Work out the finished part from the listing and answer in its coordinate system (mm). A direction names the side the tool comes from. Round coordinates to 2 decimals unless told otherwise and drop trailing zeros. Loops run counter-clockwise (first coordinate to the right, second up) from the corner with the lowest first, then second, coordinate; pieces in that order, holes last.
```python
from build123d import *

# Parameters (mm, degrees)
ESQUISSE1_R             = 12.5
BOSS_EXTRU_1_DEPTH      = 25
BOSS_EXTRU_2_DEPTH      = 40
CONG_1_R                = 10
ESQUISSE5_W             = 15
ESQUISSE5_H             = 25
BOSS_EXTRU_3_DEPTH      = 50
BOSS_EXTRU_4_DEPTH      = 5
BOSS_EXTRU_4_DEPTH_BACK = 35
ESQUISSE6_W             = 40
ESQUISSE6_H             = 40
CONG_2_R                = 10
CONG_3_R                = 10
ESQUISSE8_R             = 7.5
ENL_V_MAT_EXTRU_2_DEPTH = 20
CONG_4_R                = 10


with BuildPart() as part:
    # Esquisse1 → Boss.-Extru.1 (new body)
    with BuildSketch(Plane.XY):
        Circle(ESQUISSE1_R)
    extrude(amount=BOSS_EXTRU_1_DEPTH)

    # Esquisse2 → Boss.-Extru.2 (add)
    with BuildSketch(Plane.XY.offset(25)):
        with BuildLine():
            Line((-10, 20), (10, 20))
            ThreePointArc((10, 20), (17.071067812, 17.071067812), (20, 10))
            Line((20, 10), (20, -10))
            ThreePointArc((20, -10), (17.071067812, -17.071067812), (10, -20))
            Line((10, -20), (-10, -20))
            ThreePointArc((-10, -20), (-17.071067812, -17.071067812), (-20, -10))
            Line((-20, -10), (-20, 10))
            ThreePointArc((-20, 10), (-17.071067812, 17.071067812), (-10, 20))
        make_face()
    extrude(amount=BOSS_EXTRU_2_DEPTH)

    # Congé1
    cong_1_edges = [part.edges().sort_by_distance(p)[0] for p in [
        (0, 20, 65),
        (-17.071067812, 17.071067812, 65),
        (-20, 0, 65),
        (-17.071067812, -17.071067812, 65),
        (0, -20, 65),
        (17.071067812, -17.071067812, 65),
        (20, 0, 65),
        (17.071067812, 17.071067812, 65),
    ]]
    fillet(cong_1_edges, radius=CONG_1_R)

    # Esquisse5 → Boss.-Extru.3 (add)
    with BuildSketch(Plane.XZ.offset(20)):
        with Locations((0, 40)):
            Rectangle(ESQUISSE5_W, ESQUISSE5_H)
    extrude(amount=BOSS_EXTRU_3_DEPTH)

    # Esquisse6 → Boss.-Extru.4 (add, two sides: drawn at the far end of the back side and taken through both)
    with BuildSketch(Plane(origin=(0, 0, 27.5), x_dir=(-1, 0, 0), z_dir=(0, 0, -1)).offset(-BOSS_EXTRU_4_DEPTH_BACK)):
        with Locations((0, -90)):
            Rectangle(ESQUISSE6_W, ESQUISSE6_H)
    extrude(amount=BOSS_EXTRU_4_DEPTH + BOSS_EXTRU_4_DEPTH_BACK)

    # Congé2
    cong_2_edges = [part.edges().sort_by_distance(p)[0] for p in [
        (-20, -110, 42.5),
        (0, -110, 62.5),
        (20, -110, 42.5),
        (0, -110, 22.5),
    ]]
    fillet(cong_2_edges, radius=CONG_2_R)

    # Congé3
    # the kernel refuses this fillet: 10 mm, written as the material it takes off along each edge
    with BuildSketch(Plane(origin=(10, -100, 32.5), x_dir=(1, 0, 0), z_dir=(0, 0, -1))) as cong_3_piece_1_section:
        Polygon((0, 0), (CONG_3_R, 0), (CONG_3_R, CONG_3_R), (0, CONG_3_R), align=None)
    cong_3_piece_1 = extrude(amount=CONG_3_R, mode=Mode.PRIVATE)
    cong_3_piece_1 = cong_3_piece_1 - Plane(origin=(10, -100, 32.5), x_dir=(-0.7071067811865475, 0.7071067811865475, 0), z_dir=(0, 0, -1)) * Sphere(CONG_3_R, mode=Mode.PRIVATE)
    add(cong_3_piece_1, mode=Mode.SUBTRACT)
    with BuildSketch(Plane(origin=(-10, -100, 32.5), x_dir=(0, 0, -1), z_dir=(-1, 0, 0))) as cong_3_piece_2_section:
        Polygon((0, 0), (CONG_3_R, 0), (CONG_3_R, CONG_3_R), (0, CONG_3_R), align=None)
    cong_3_piece_2 = extrude(amount=CONG_3_R, mode=Mode.PRIVATE)
    cong_3_piece_2 = cong_3_piece_2 - Plane(origin=(-10, -100, 32.5), x_dir=(0, 0.7071067811865475, 0.7071067811865475), z_dir=(-1, 0, 0)) * Sphere(CONG_3_R, mode=Mode.PRIVATE)
    add(cong_3_piece_2, mode=Mode.SUBTRACT)
    with BuildSketch(Plane(origin=(10, -100, 52.5), x_dir=(1, 0, 0), z_dir=(0, 0, 1))) as cong_3_piece_3_section:
        Polygon((0, 0), (CONG_3_R, 0), (CONG_3_R, -CONG_3_R), (0, -CONG_3_R), align=None)
    cong_3_piece_3 = extrude(amount=CONG_3_R, mode=Mode.PRIVATE)
    cong_3_piece_3 = cong_3_piece_3 - Plane(origin=(10, -100, 52.5), x_dir=(-0.7071067811865475, 0.7071067811865475, 0), z_dir=(0, 0, 1)) * Sphere(CONG_3_R, mode=Mode.PRIVATE)
    add(cong_3_piece_3, mode=Mode.SUBTRACT)
    with BuildSketch(Plane(origin=(-10, -100, 52.5), x_dir=(0, 0, 1), z_dir=(-1, 0, 0))) as cong_3_piece_4_section:
        Polygon((0, 0), (CONG_3_R, 0), (CONG_3_R, -CONG_3_R), (0, -CONG_3_R), align=None)
    cong_3_piece_4 = extrude(amount=CONG_3_R, mode=Mode.PRIVATE)
    cong_3_piece_4 = cong_3_piece_4 - Plane(origin=(-10, -100, 52.5), x_dir=(0, 0.7071067811865475, -0.7071067811865475), z_dir=(-1, 0, 0)) * Sphere(CONG_3_R, mode=Mode.PRIVATE)
    add(cong_3_piece_4, mode=Mode.SUBTRACT)
    with BuildSketch(Plane(origin=(20, -45, 62.5), x_dir=(-1, 0, 0), z_dir=(0, -1, 0)), Plane(origin=(-20, -100, 22.5), x_dir=(0, 0, 1), z_dir=(0, 1, 0))) as cong_3_piece_5:
        with BuildLine():
            CenterArc((CONG_3_R, CONG_3_R), CONG_3_R, 180, 90)
            Line((0, CONG_3_R), (0, 0))
            Line((0, 0), (CONG_3_R, 0))
        make_face()
    extrude(amount=55, mode=Mode.SUBTRACT)
    with BuildSketch(Plane(origin=(20, -45, 22.5), x_dir=(-1, 0, 0), z_dir=(0, -1, 0)), Plane(origin=(-20, -100, 62.5), x_dir=(0, 0, -1), z_dir=(0, 1, 0))) as cong_3_piece_6:
        with BuildLine():
            CenterArc((CONG_3_R, -CONG_3_R), CONG_3_R, 90, 90)
            Line((0, -CONG_3_R), (0, 0))
            Line((0, 0), (CONG_3_R, 0))
        make_face()
    extrude(amount=55, mode=Mode.SUBTRACT)

    # Esquisse8 → Enlèv. mat.-Extru.2 (cut)
    with BuildSketch(Plane(origin=(0, 0, 22.5), x_dir=(-1, 0, 0), z_dir=(0, 0, -1))):
        with Locations((0, -85)):
            Circle(ESQUISSE8_R)
    extrude(amount=-ENL_V_MAT_EXTRU_2_DEPTH, mode=Mode.SUBTRACT)

    # Congé4
    # the kernel refuses this fillet: 10 mm, written as the material it takes off along each edge
    with BuildSketch(Plane(origin=(-10, -70, 52.5), x_dir=(0, 0, 1), z_dir=(1, 0, 0))) as cong_4_piece_1:
        with BuildLine():
            CenterArc((10 - CONG_4_R, CONG_4_R), CONG_4_R, 270, 90)
            Line((10 - CONG_4_R, 0), (10, 0))
            Line((10, 0), (10, CONG_4_R))
        make_face()
    revolve(axis=Axis((-10, -70, 52.5), (0, -1, 0)), revolution_arc=90, mode=Mode.SUBTRACT)
    with BuildSketch(Plane(origin=(-10, -70, 62.5), x_dir=(0, 0, -1), z_dir=(1, 0, 0)), Plane(origin=(20, -70, 52.5), x_dir=(-1, 0, 0), z_dir=(0, 0, -1))) as cong_4_piece_2:
        with BuildLine():
            CenterArc((CONG_4_R, -CONG_4_R), CONG_4_R, 90, 90)
            Line((0, -CONG_4_R), (0, 0))
            Line((0, 0), (CONG_4_R, 0))
        make_face()
    extrude(amount=20, mode=Mode.SUBTRACT)
    with BuildSketch(Plane(origin=(10, -70, 52.5), x_dir=(0, 0, 1), z_dir=(-1, 0, 0))) as cong_4_piece_3:
        with BuildLine():
            CenterArc((10 - CONG_4_R, -CONG_4_R), CONG_4_R, 0, 90)
            Line((10, -CONG_4_R), (10, 0))
            Line((10, 0), (10 - CONG_4_R, 0))
        make_face()
    revolve(axis=Axis((10, -70, 52.5), (0, 1, 0)), revolution_arc=90, mode=Mode.SUBTRACT)
    with BuildSketch(Plane(origin=(10, -70, 32.5), x_dir=(1, 0, 0), z_dir=(0, 0, 1))) as cong_4_piece_4:
        with BuildLine():
            CenterArc((10 - CONG_4_R, -CONG_4_R), CONG_4_R, 0, 90)
            Line((10, -CONG_4_R), (10, 0))
            Line((10, 0), (10 - CONG_4_R, 0))
        make_face()
    revolve(axis=Axis((10, -70, 32.5), (0, 1, 0)), revolution_arc=90, mode=Mode.SUBTRACT)
    with BuildSketch(Plane(origin=(-10, -70, 22.5), x_dir=(0, 0, 1), z_dir=(1, 0, 0))) as cong_4_piece_5_section:
        with BuildLine():
            CenterArc((CONG_4_R, CONG_4_R), CONG_4_R, 180, 90)
            Line((0, CONG_4_R), (0, 0))
            Line((0, 0), (CONG_4_R, 0))
        make_face()
    cong_4_piece_5 = extrude(amount=20, mode=Mode.PRIVATE)
    cong_4_piece_5 = split(cong_4_piece_5, bisect_by=Plane(origin=(-8.75, -70.240083817, 27.5), z_dir=(0, 0, 1)), keep=Keep.TOP, mode=Mode.PRIVATE)
    cong_4_piece_5 = split(cong_4_piece_5, bisect_by=Plane(origin=(-7.5, -70.240083817, 29.132507845), z_dir=(-1, 0, 0)), keep=Keep.TOP, mode=Mode.PRIVATE)
    add(cong_4_piece_5, mode=Mode.SUBTRACT)
    with BuildSketch(Plane(origin=(-10, -70, 22.5), x_dir=(0, 0, 1), z_dir=(1, 0, 0))) as cong_4_piece_6_section:
        with BuildLine():
            CenterArc((CONG_4_R, CONG_4_R), CONG_4_R, 180, 90)
            Line((0, CONG_4_R), (0, 0))
            Line((0, 0), (CONG_4_R, 0))
        make_face()
    cong_4_piece_6 = extrude(amount=20, mode=Mode.PRIVATE)
    cong_4_piece_6 = split(cong_4_piece_6, bisect_by=Plane(origin=(-8.75, -72.5512006, 27.5), z_dir=(0, 0, -1)), keep=Keep.TOP, mode=Mode.PRIVATE)
    cong_4_piece_6 = split(cong_4_piece_6, bisect_by=Plane(origin=(-7.5, -72.5512006, 24.143917643), z_dir=(-1, 0, 0)), keep=Keep.TOP, mode=Mode.PRIVATE)
    add(cong_4_piece_6, mode=Mode.SUBTRACT)
    with BuildSketch(Plane(origin=(-10, -70, 22.5), x_dir=(0, 0, 1), z_dir=(1, 0, 0))) as cong_4_piece_7_section:
        with BuildLine():
            CenterArc((CONG_4_R, CONG_4_R), CONG_4_R, 180, 90)
            Line((0, CONG_4_R), (0, 0))
            Line((0, 0), (CONG_4_R, 0))
        make_face()
    cong_4_piece_7 = extrude(amount=20, mode=Mode.PRIVATE)
    cong_4_piece_7 = split(cong_4_piece_7, bisect_by=Plane(origin=(0, -72.5512006, 27.5), z_dir=(0, 0, -1)), keep=Keep.TOP, mode=Mode.PRIVATE)
    cong_4_piece_7 = split(cong_4_piece_7, bisect_by=Plane(origin=(7.5, -72.5512006, 24.143917643), z_dir=(-1, 0, 0)), keep=Keep.TOP, mode=Mode.PRIVATE)
    cong_4_piece_7 = split(cong_4_piece_7, bisect_by=Plane(origin=(-7.5, -72.5512006, 24.143917643), z_dir=(1, 0, 0)), keep=Keep.TOP, mode=Mode.PRIVATE)
    add(cong_4_piece_7, mode=Mode.SUBTRACT)
    with BuildSketch(Plane(origin=(-10, -70, 22.5), x_dir=(0, 0, 1), z_dir=(1, 0, 0))) as cong_4_piece_8_section:
        with BuildLine():
            CenterArc((CONG_4_R, CONG_4_R), CONG_4_R, 180, 90)
            Line((0, CONG_4_R), (0, 0))
            Line((0, 0), (CONG_4_R, 0))
        make_face()
    cong_4_piece_8 = extrude(amount=20, mode=Mode.PRIVATE)
    cong_4_piece_8 = split(cong_4_piece_8, bisect_by=Plane(origin=(8.75, -70.240083817, 27.5), z_dir=(0, 0, 1)), keep=Keep.TOP, mode=Mode.PRIVATE)
    cong_4_piece_8 = split(cong_4_piece_8, bisect_by=Plane(origin=(7.5, -70.240083817, 29.132507845), z_dir=(1, 0, 0)), keep=Keep.TOP, mode=Mode.PRIVATE)
    add(cong_4_piece_8, mode=Mode.SUBTRACT)
    with BuildSketch(Plane(origin=(-10, -70, 22.5), x_dir=(0, 0, 1), z_dir=(1, 0, 0))) as cong_4_piece_9_section:
        with BuildLine():
            CenterArc((CONG_4_R, CONG_4_R), CONG_4_R, 180, 90)
            Line((0, CONG_4_R), (0, 0))
            Line((0, 0), (CONG_4_R, 0))
        make_face()
    cong_4_piece_9 = extrude(amount=20, mode=Mode.PRIVATE)
    cong_4_piece_9 = split(cong_4_piece_9, bisect_by=Plane(origin=(8.75, -72.5512006, 27.5), z_dir=(0, 0, -1)), keep=Keep.TOP, mode=Mode.PRIVATE)
    cong_4_piece_9 = split(cong_4_piece_9, bisect_by=Plane(origin=(7.5, -72.5512006, 24.143917643), z_dir=(1, 0, 0)), keep=Keep.TOP, mode=Mode.PRIVATE)
    add(cong_4_piece_9, mode=Mode.SUBTRACT)
    with BuildSketch(Plane(origin=(-10, -70, 32.5), x_dir=(-1, 0, 0), z_dir=(0, 0, 1))) as cong_4_piece_10:
        with BuildLine():
            CenterArc((10 - CONG_4_R, CONG_4_R), CONG_4_R, 270, 90)
            Line((10, CONG_4_R), (10, 0))
            Line((10, 0), (10 - CONG_4_R, 0))
        make_face()
    revolve(axis=Axis((-10, -70, 32.5), (0, -1, 0)), revolution_arc=90, mode=Mode.SUBTRACT)
    with BuildSketch(Plane(origin=(-20, -70, 32.5), x_dir=(0, -1, 0), z_dir=(0, 0, 1))) as cong_4_piece_11:
        with BuildLine():
            CenterArc((CONG_4_R, CONG_4_R), CONG_4_R, 180, 90)
            Line((0, CONG_4_R), (0, 0))
            Line((0, 0), (CONG_4_R, 0))
        make_face()
    extrude(amount=20, mode=Mode.SUBTRACT)


solid = part.part
```
1. Given pin 1 (22 mm diameter, centred on x = 0.5, y = -93.5, fed in from -Z); pin 2 (13.5 mm diameter, centred on x = 0, y = -85, fed in from +Z); pin 3 (4.5 mm diameter, centred on x = -3, y = -50.5, fed in from -Z); pin 4 (20 mm diameter, centred on x = -2, y = -5, fed in from -Z), each flat-ended and moving along its own axis, determine where each tip first touches the part or whether it passes through.
Answer key:
pin 1: stops at z = 22.5
pin 2: stops at z = 62.5
pin 3: stops at z = 27.5
pin 4: stops at z = 0
2. Which of the six approach directions +Z, -Z, +X, -X, +Y, -Y give full straight-line access (tool end or side, diameter ignored) to faces 4 (the face through (17.15, -16.99, 39.79)), 5 (the face through (11.923, 3.755, 12.325)), 6 (the face through (16.99, -89.86, 25.35)), 7 (the face through (-16.99, -90.14, 25.35)), 8 (the face through (-0.14, -72.85, 59.49))?
Answer key:
face 4: +Z, -Z, +X
face 5: -Z
face 6: -Z, +X, -Y
face 7: -Z, -X, -Y
face 8: +Z, +X, -X
3. Find section C-C (x = 14.5). Write down the section's boundary in (y, z), then the cut area to 3 significant figures.
Answer key:
outline: (-108.93, 32.5) arc R8.93 ccw to (-100, 23.57) - (-80, 23.57) arc R8.93 ccw to (-71.07, 32.5) - (-71.07, 52.5) arc R8.93 ccw to (-80, 61.43) - (-100, 61.43) arc R8.93 ccw to (-108.93, 52.5) - close; (-18.93, 25) - (18.93, 25) - (18.93, 55) arc R8.93 ccw to (10, 63.93) - (-10, 63.93) arc R8.93 ccw to (-18.93, 55) - close
area: 2,800 mm2
4. Find section A-A (x = -16). Write down the section's boundary in (y, z), then the cut area to 3 significant figures.
Answer key:
outline: (-108, 32.5) arc R8 ccw to (-100, 24.5) - (-80, 24.5) arc R8 ccw to (-72, 32.5) - (-72, 52.5) arc R8 ccw to (-80, 60.5) - (-100, 60.5) arc R8 ccw to (-108, 52.5) - close; (-18, 25) - (18, 25) - (18, 55) arc R8 ccw to (10, 63) - (-10, 63) arc R8 ccw to (-18, 55) - close
area: 2,580 mm2
5. Consider probe 1 along Y at (x, z) = (8, 40.5); probe 2 along Y at (x, z) = (0, 27); probe 3 along X at (y, z) = (-85, 35.75). Determine where each line is inside the solid, lowest interval first.
Answer key:
probe 1: y = -110 to -70, -20 to 20
probe 2: y = -108.35 to -92.5, -77.5 to -71.65, -20 to 20
probe 3: x = -20 to -7.5, 7.5 to 20
6. Determine the mould class of faces 1 (the face through (-20, 0, 40)), 2 (the face through (-9, -70, 43)), 3 (the face through (0.14, 17.15, 61.99)) for opening direction Y: +Y half, -Y half, draft (parallel to the pull), parting line (faces both ways), or undercut.
Answer key:
face 1: draft
face 2: undercut
face 3: +Y half
7. Find section B-B (y = -85). Write down the section's boundary in (x, z), then the cut area to 3 significant figures.
Answer key:
outline: (-20, 32.5) arc R10 ccw to (-10, 22.5) - (-7.5, 22.5) - (-7.5, 42.5) - (7.5, 42.5) - (7.5, 22.5) - (10, 22.5) arc R10 ccw to (20, 32.5) - (20, 52.5) arc R10 ccw to (10, 62.5) - (-10, 62.5) arc R10 ccw to (-20, 52.5) - close
area: 1,210 mm2
8. Find section D-D (z = 6). Write down the section's boundary in (x, y).
Answer key:
outline: circle Ø25 at (0, 0)
